Job drawing, mm, ordinate dimensions from the low corner. One solid piece. A direction names the side the tool comes from. Give positions to 0.01 mm unless a question says otherwise; leave off trailing zeros. Order: outer loops, then holes, each group sorted by start corner. A loop starts at its lowest first (then second) coordinate and runs counter-clockwise, first axis right, second up. Notation, with made-up numbers: M 52,16.5 L 59,16.5 A31 cw 59,52.5 Z; hole C 75,-18.75 d7. An arc over 180 degrees is marked long. Use CSV: the item, a comma, the result in double quotes. Start each with the question number.
Item 1: Band-saw the part on C-C on z = 12.7. Give the number of separate pieces and of enclosed holes in the cut face.
Item 2: Pin check, flat tip, straight feed: P1, Ø5, axis at x = 20, z = 5, coming from the +Y side. Stop position of the tip, or through.
Item 3: Two-plate mould, pull along Z, no slides. Class the marked faces 3, 4 and 5: pulls with the +Z half, pulls with the -Z half, needs draft (parallel to the pull), parting line crosses it, or undercut.
Item 4: Band-saw the part on D-D on y = 93.5. Write the cut outline in (x, z), plus the area to 3 significant figures.
Item 5: Which spindle directions (+Z, -Z, +X, -X, +Y, -Y) get a long thin tool onto all of the face, cutting with end or side? Do the marked faces 1 and 2. Say none if no direction does.
Item 6: Wall check: line 1 along X through (y, z) = (120, 20.75); line 2 along Z through (x, y) = (7.5, 63); line 3 along Z through (x, y) = (50.1, 165.1). Give the ranges that are in metal, low to high.
Item 7: Band-saw the part on A-A on x = 42.5. Write the cut outline in (y, z).
Item 8: Band-saw the part on B-B on y = 171.45. Write the cut outline in (x, z).
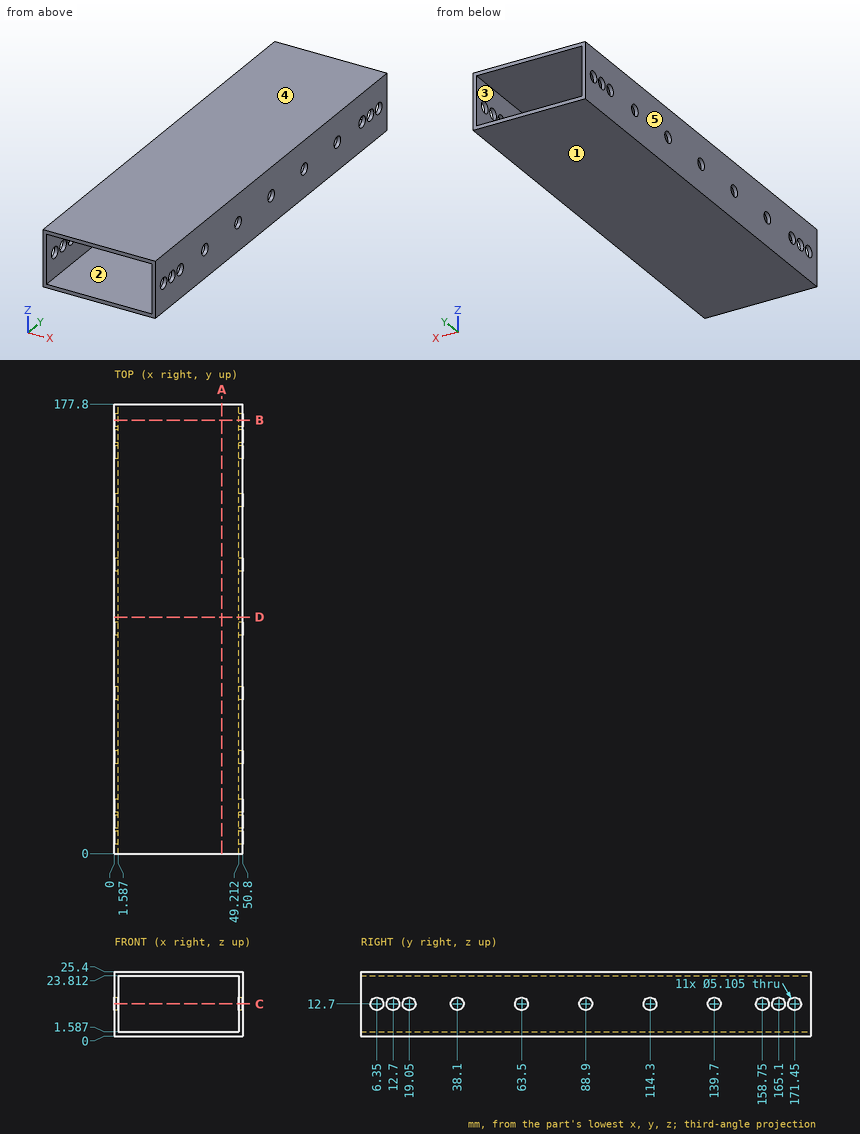
Model answer:
1,separate pieces,"24"
1,enclosed holes,"0"
2,P1,"passes through"
3,face 3,"undercut"
3,face 4,"pulls with the +Z half"
3,face 5,"needs draft"
4,outline,"M 0,0 L 50.8,0 L 50.8,25.4 L 0,25.4 Z; hole M 1.59,1.59 L 49.21,1.59 L 49.21,23.81 L 1.59,23.81 Z"
4,area,"232 mm^2"
5,face 1,"-Z, +X, -X, +Y, -Y"
5,face 2,"+Y, -Y"
6,line 1,"x = 0 to 1.59, 49.21 to 50.8"
6,line 2,"z = 0 to 1.59, 23.81 to 25.4"
6,line 3,"z = 0 to 10.15, 15.25 to 25.4"
7,outline,"M 0,0 L 177.8,0 L 177.8,1.59 L 0,1.59 Z; M 0,23.81 L 177.8,23.81 L 177.8,25.4 L 0,25.4 Z"
8,outline,"M 0,0 L 50.8,0 L 50.8,10.15 L 49.21,10.15 L 49.21,1.59 L 1.59,1.59 L 1.59,10.15 L 0,10.15 Z; M 0,15.25 L 1.59,15.25 L 1.59,23.81 L 49.21,23.81 L 49.21,15.25 L 50.8,15.25 L 50.8,25.4 L 0,25.4 Z"
